```python
from build123d import *

# Parameters (mm, degrees)
BOSS_EXTRUDE2_DEPTH             = 20
CUT_EXTRUDE1_START              = -9.5
CUT_EXTRUDE1_DEPTH              = 9.5
CBORE_FOR_M4_SHCS1_D            = 4.5
CBORE_FOR_M4_SHCS1_CBORE_D      = 8
CBORE_FOR_M4_SHCS1_CBORE_DEPTH  = 4
CUT_EXTRUDE2_DEPTH              = 12
CUT_EXTRUDE3_DEPTH              = 69.381283989
CUT_EXTRUDE3_DEPTH_BACK         = 69.381283989
CBORE_START                     = 12
CBORE_SLOT_FOR_M3_SHCS1_DEPTH   = 8
CBORE_SLOT_FOR_M3_SHCS1_2_DEPTH = 3
CUT_EXTRUDE4_DEPTH              = 10
CUT_EXTRUDE4_DEPTH_BACK         = 111.48189897
M14_CLEARANCE_HOLE1_D           = 15.5
CBORE_FOR_M4_SHCS2_D            = 4.5
CBORE_FOR_M4_SHCS2_CBORE_D      = 8
CBORE_FOR_M4_SHCS2_CBORE_DEPTH  = 4
BOSS_EXTRUDE3_REACH             = 70.381
SKETCH16_W                      = 17
SKETCH16_H                      = 5.63508794
CUT_EXTRUDE5_DEPTH              = 69.381284106
CUT_EXTRUDE5_DEPTH_BACK         = 69.381284106
SKETCH18_W                      = 14.5
SKETCH18_H                      = 5.25


# Read off the part's stored shape, not the designer's step: CBORE SLOT for M3 SHCS1
with BuildPart() as part:
    # Sketch2 → Boss-Extrude2 (new body)
    with BuildSketch(Plane.XY):
        with BuildLine():
            Line((54, 26), (-47.5, 26))
            ThreePointArc((-47.5, 26), (-56.338834765, 22.338834765), (-60, 13.5))
            Line((-60, 13.5), (-60, -13.5))
            ThreePointArc((-60, -13.5), (-56.338834765, -22.338834765), (-47.5, -26))
            Line((-47.5, -26), (54, -26))
            ThreePointArc((54, -26), (58.242640687, -24.242640687), (60, -20))
            Line((60, -20), (60, 20))
            ThreePointArc((60, 20), (58.242640687, 24.242640687), (54, 26))
        make_face()
    extrude(amount=BOSS_EXTRUDE2_DEPTH)

    # Sketch3 → Cut-Extrude1 (cut)
    with BuildSketch(Plane.XY.offset(20).offset(CUT_EXTRUDE1_START)):
        with BuildLine():
            Line((-47.5, -26), (-24, -26))
            Line((-24, -26), (-24, -17))
            ThreePointArc((-24, -17), (-25.464466094, -13.464466094), (-29, -12))
            Line((-29, -12), (-45.5, -12))
            Line((-45.5, -12), (-45.5, 12))
            Line((-45.5, 12), (-29, 12))
            ThreePointArc((-29, 12), (-25.464466094, 13.464466094), (-24, 17))
            Line((-24, 17), (-24, 26))
            Line((-24, 26), (-47.5, 26))
            ThreePointArc((-47.5, 26), (-56.338834765, 22.338834765), (-60, 13.5))
            Line((-60, 13.5), (-60, -13.5))
            ThreePointArc((-60, -13.5), (-56.338834765, -22.338834765), (-47.5, -26))
        make_face()
        with BuildLine():
            Line((39, 12), (60, 12))
            Line((60, 12), (60, 20))
            ThreePointArc((60, 20), (58.242640687, 24.242640687), (54, 26))
            Line((54, 26), (34, 26))
            Line((34, 26), (34, 17))
            ThreePointArc((34, 17), (35.464466094, 13.464466094), (39, 12))
        make_face()
        with BuildLine():
            Line((60, -20), (60, -12))
            Line((60, -12), (39, -12))
            ThreePointArc((39, -12), (35.464466094, -13.464466094), (34, -17))
            Line((34, -17), (34, -26))
            Line((34, -26), (54, -26))
            ThreePointArc((54, -26), (58.242640687, -24.242640687), (60, -20))
        make_face()
    extrude(amount=CUT_EXTRUDE1_DEPTH, mode=Mode.SUBTRACT)

    # CBORE for M4 SHCS1 (through all)
    with Locations(Plane.XY.offset(10.5)):
        with Locations((39, -17), (39, 17), (-29, 17), (-29, -17), (54, 20), (54, -20)):
            CounterBoreHole(CBORE_FOR_M4_SHCS1_D / 2, CBORE_FOR_M4_SHCS1_CBORE_D / 2, CBORE_FOR_M4_SHCS1_CBORE_DEPTH)

    # Sketch6 → Cut-Extrude2 (cut)
    with BuildSketch(Plane.XY):
        with BuildLine():
            Line((25, -21), (-15, -21))
            ThreePointArc((-15, -21), (-18.535533906, -19.535533906), (-20, -16))
            Line((-20, -16), (-20, 16))
            ThreePointArc((-20, 16), (-18.535533906, 19.535533906), (-15, 21))
            Line((-15, 21), (25, 21))
            ThreePointArc((25, 21), (28.535533906, 19.535533906), (30, 16))
            Line((30, 16), (30, -16))
            ThreePointArc((30, -16), (28.535533906, -19.535533906), (25, -21))
        make_face()
    extrude(amount=CUT_EXTRUDE2_DEPTH, mode=Mode.SUBTRACT)

    # Sketch7 → Cut-Extrude3 (cut, two sides: drawn at the far end of the back side and taken through both)
    with BuildSketch(Plane(origin=(0, 0, 0), x_dir=(1, 0, 0), z_dir=(0, 1, 0)).offset(-CUT_EXTRUDE3_DEPTH_BACK)):
        Polygon((-12.5, 0), (22.5, 0), (17.881197846, -8), (-7.881197846, -8), align=None)
    extrude(amount=CUT_EXTRUDE3_DEPTH + CUT_EXTRUDE3_DEPTH_BACK, mode=Mode.SUBTRACT)

    # CBORE SLOT for M3 SHCS1 outline → CBORE SLOT for M3 SHCS1 (cut)
    with BuildSketch(Plane.XY.offset(CBORE_START)):
        with BuildLine():
            ThreePointArc((-8.717871555, 16.122034611), (-11.122034611, 16.122034611), (-11.122034611, 13.717871555))
            Line((-11.122034611, 13.717871555), (-5.040916293, 7.636753237))
            ThreePointArc((-5.040916293, 7.636753237), (-2.636753237, 7.636753237), (-2.636753237, 10.040916293))
            Line((-2.636753237, 10.040916293), (-8.717871555, 16.122034611))
        make_face()
        with BuildLine():
            ThreePointArc((18.717871555, -16.122034611), (21.122034611, -16.122034611), (21.122034611, -13.717871555))
            Line((21.122034611, -13.717871555), (15.040916293, -7.636753237))
            ThreePointArc((15.040916293, -7.636753237), (12.636753237, -7.636753237), (12.636753237, -10.040916293))
            Line((12.636753237, -10.040916293), (18.717871555, -16.122034611))
        make_face()
    cbore_slot_for_m3_shcs1 = extrude(amount=CBORE_SLOT_FOR_M3_SHCS1_DEPTH, mode=Mode.SUBTRACT)

    # CBORE SLOT for M3 SHCS1 2 outline → CBORE SLOT for M3 SHCS1 2 (cut)
    # profile 1 of 2: a face of its own
    with BuildSketch(Plane.XY.offset(CBORE_START)):
        with BuildLine():
            ThreePointArc((-7.621856044, 17.218050122), (-12.218050122, 17.218050122), (-12.218050122, 12.621856044))
            Line((-12.218050122, 12.621856044), (-6.136931804, 6.540737726))
            ThreePointArc((-6.136931804, 6.540737726), (-1.540737726, 6.540737726), (-1.540737726, 11.136931804))
            Line((-1.540737726, 11.136931804), (-7.621856044, 17.218050122))
        make_face()
        with BuildLine():
            Line((-5.040916293, 7.636753237), (-11.122034611, 13.717871555))
            ThreePointArc((-11.122034611, 13.717871555), (-11.122034611, 16.122034611), (-8.717871555, 16.122034611))
            Line((-8.717871555, 16.122034611), (-2.636753237, 10.040916293))
            ThreePointArc((-2.636753237, 10.040916293), (-2.636753237, 7.636753237), (-5.040916293, 7.636753237))
        make_face(mode=Mode.SUBTRACT)
    # profile 2 of 2: a face of its own
    with BuildSketch(Plane.XY.offset(CBORE_START)):
        with BuildLine():
            ThreePointArc((17.621856044, -17.218050122), (22.218050122, -17.218050122), (22.218050122, -12.621856044))
            Line((22.218050122, -12.621856044), (16.136931804, -6.540737726))
            ThreePointArc((16.136931804, -6.540737726), (11.540737726, -6.540737726), (11.540737726, -11.136931804))
            Line((11.540737726, -11.136931804), (17.621856044, -17.218050122))
        make_face()
        with BuildLine():
            Line((15.040916293, -7.636753237), (21.122034611, -13.717871555))
            ThreePointArc((21.122034611, -13.717871555), (21.122034611, -16.122034611), (18.717871555, -16.122034611))
            Line((18.717871555, -16.122034611), (12.636753237, -10.040916293))
            ThreePointArc((12.636753237, -10.040916293), (12.636753237, -7.636753237), (15.040916293, -7.636753237))
        make_face(mode=Mode.SUBTRACT)
    cbore_slot_for_m3_shcs1_2 = extrude(amount=CBORE_SLOT_FOR_M3_SHCS1_2_DEPTH, mode=Mode.SUBTRACT)

    # Mirror1: CBORE SLOT for M3 SHCS1, CBORE SLOT for M3 SHCS1 2 across plane
    add(cbore_slot_for_m3_shcs1.mirror(Plane.ZX), mode=Mode.SUBTRACT)
    add(cbore_slot_for_m3_shcs1_2.mirror(Plane.ZX), mode=Mode.SUBTRACT)

    # Sketch10 → Cut-Extrude4 (cut, two sides: drawn at the far end of the back side and taken through both)
    with BuildSketch(Plane.ZY.offset(45.5).offset(-CUT_EXTRUDE4_DEPTH_BACK)):
        with BuildLine():
            Line((0, 12.6), (0, -12.6))
            ThreePointArc((0, -12.6), (12.6, 0), (0, 12.6))
        make_face()
    extrude(amount=CUT_EXTRUDE4_DEPTH + CUT_EXTRUDE4_DEPTH_BACK, mode=Mode.SUBTRACT)

    # M14 Clearance Hole1 (through all)
    with Locations(Plane.XY.offset(20)):
        with Locations((5, 0)):
            Hole(M14_CLEARANCE_HOLE1_D / 2)

    # CBORE for M4 SHCS2 (through all)
    with Locations(Plane.XY.offset(20)):
        with Locations((49.5, 0)):
            CounterBoreHole(CBORE_FOR_M4_SHCS2_D / 2, CBORE_FOR_M4_SHCS2_CBORE_D / 2, CBORE_FOR_M4_SHCS2_CBORE_DEPTH)

    # Sketch16 → Boss-Extrude3 (add, up to next)
    with BuildSketch(Plane(origin=(0, 0, 0), x_dir=(-1, 0, 0), z_dir=(0, 0, -1)), mode=Mode.PRIVATE) as boss_extrude3_sk1:
        with Locations((47, 9.78245603)):
            Rectangle(SKETCH16_W, SKETCH16_H)
    boss_extrude3_tool1 = extrude(boss_extrude3_sk1.sketch, amount=-BOSS_EXTRUDE3_REACH, mode=Mode.PRIVATE) - part.part
    # Sketch16 → Boss-Extrude3 (add, up to next)
    with BuildSketch(Plane(origin=(0, 0, 0), x_dir=(-1, 0, 0), z_dir=(0, 0, -1)), mode=Mode.PRIVATE) as boss_extrude3_sk2:
        with Locations((47, -9.78245603)):
            Rectangle(SKETCH16_W, SKETCH16_H)
    boss_extrude3_tool2 = extrude(boss_extrude3_sk2.sketch, amount=-BOSS_EXTRUDE3_REACH, mode=Mode.PRIVATE) - part.part
    add(boss_extrude3_tool1.solids().sort_by_distance((-47, 9.782456, 0))[0])
    add(boss_extrude3_tool2.solids().sort_by_distance((-47, -9.782456, 0))[0])

    # Sketch18 → Cut-Extrude5 (cut, two sides: drawn at the far end of the back side and taken through both)
    with BuildSketch(Plane(origin=(0, 0, 0), x_dir=(1, 0, 0), z_dir=(0, 1, 0)).offset(-CUT_EXTRUDE5_DEPTH_BACK)):
        with Locations((-52.75, -2.625)):
            Rectangle(SKETCH18_W, SKETCH18_H)
    extrude(amount=CUT_EXTRUDE5_DEPTH + CUT_EXTRUDE5_DEPTH_BACK, mode=Mode.SUBTRACT)


solid = part.part
```
Work out the finished part from the listing and answer in its coordinate system (mm). A direction names the side the tool comes from. Coordinates: 2 decimals unless noted, no trailing zeros. Write each loop counter-clockwise with the first axis right and the second up, starting at its lowest first coordinate (ties: lowest second). Pieces come first, ordered by that corner, then holes. Notation, with made-up numbers: (-1.5, -30) - (45.5, -30) arc R20 ccw to (45.5, -18) - close; hole circle Ø7 at (56.25, 35). An arc over 180 degrees is marked (long way). Answer as a JSON object with one key per item and string values.
Q1. Which of the six approach directions +Z, -Z, +X, -X, +Y, -Y give full straight-line access (tool end or side, diameter ignored) to faces 4 (the cylindrical face through (45.504, 0.176, 18.028)), 5 (the flat face through (5, -21, 9)), 6 (the flat face through (20.223, -23.535, 3.944)), 7 (the flat face through (49, 12, 15)), 8 (the flat face through (15.635, -13.039, 17.465))?
Results list:
{"face 4": "+Z", "face 5": "-Z", "face 6": "-Z, +Y, -Y", "face 7": "+Z, +X, +Y", "face 8": "+Z, -Z"}
Q2. Find section B-B (x = 5). Write down the section's boundary in (y, z), plus the area to 3 significant figures.
Results list:
{"outline": "(-26, 8) - (-21, 8) - (-21, 12) - (-7.75, 12) - (-7.75, 20) - (-26, 20) - close; (7.75, 12) - (21, 12) - (21, 8) - (26, 8) - (26, 20) - (7.75, 20) - close", "area": "332 mm^2"}
Q3. Given pin 1 Ø4 at (y, z) = (1, 2.5) entering from +X; pin 2 Ø6.5 at (x, y) = (16.5, -13) entering from -Z; pin 3 Ø3.5 at (y, z) = (7.5, 3) entering from -X; pin 4 Ø5.5 at (x, y) = (3.5, 24.5) entering from -Z, each flat-ended and moving along its own axis, determine where each tip first touches the part or whether it passes through.
Results list:
{"pin 1": "passes through", "pin 2": "stops at z = 12", "pin 3": "stops at x = -45.5", "pin 4": "stops at z = 8"}
Q4. For a pull along Y with two mould halves and no side action, classify faces 1 (the cylindrical face through (57.815, 21.201, 8.528)), 2 (the cylindrical face through (-26, 13, 15)), 3 (the cylindrical face through (-56.435, -22.241, 7.838)) as pulls with the +Y half, pulls with the -Y half, needs draft (parallel to the pull), parting line crosses it, or undercut.
Results list:
{"face 1": "undercut", "face 2": "pulls with the +Y half", "face 3": "pulls with the -Y half"}
Q5. Find section A-A (y = 0). Write down the section's boundary in (x, z).
Results list:
{"outline": "(-60, 5.25) - (-55.5, 5.25) - (-55.5, 10.5) - (-60, 10.5) - close; (-45.5, 12.6) - (-2.75, 12.6) - (-2.75, 20) - (-45.5, 20) - close; (12.75, 12.6) - (47.25, 12.6) - (47.25, 16) - (45.5, 16) - (45.5, 20) - (12.75, 20) - close; (51.75, 12.6) - (60, 12.6) - (60, 20) - (53.5, 20) - (53.5, 16) - (51.75, 16) - close"}
Q6. Consider L1, parallel to X at y = 0, z = 14.2; L2, parallel to Y at x = 49.5, z = 18.1; L3, parallel to X at y = 14, z = 18.25. Determine where each line is inside the solid, lowest interval first. Write a range as from..to.
Results list:
{"L1": "x = -45.5..-2.75, 12.75..47.25, 51.75..60", "L2": "y = -12..-4, 4..12", "L3": "x = -25..-11.35, -6.6..16.6, 21.35..35"}
Q7. Find section C-C (x = -36). Write down the section's boundary in (y, z).
Results list:
{"outline": "(-26, 0) - (-12.6, 0) arc R12.6 cw to (12.6, 0) - (26, 0) - (26, 10.5) - (12, 10.5) - (12, 20) - (-12, 20) - (-12, 10.5) - (-26, 10.5) - close"}
